The model under review builds one solid part; all positions refer to its coordinate system, in mm. Face numbers are marked on the shaded views. A direction names the side the tool comes from. Round coordinates to 2 decimals unless told otherwise and drop trailing zeros. Write each loop counter-clockwise with the first axis right and the second up, starting at its lowest first coordinate (ties: lowest second). Pieces come first, ordered by that corner, then holes. Notation, with made-up numbers: (-11, -29) - (-6, -29) arc R22 cw to (-6, 3) - close; hole circle Ø11 at (25, 5). An arc over 180 degrees is marked (long way). Use one line per item in the form item = value.
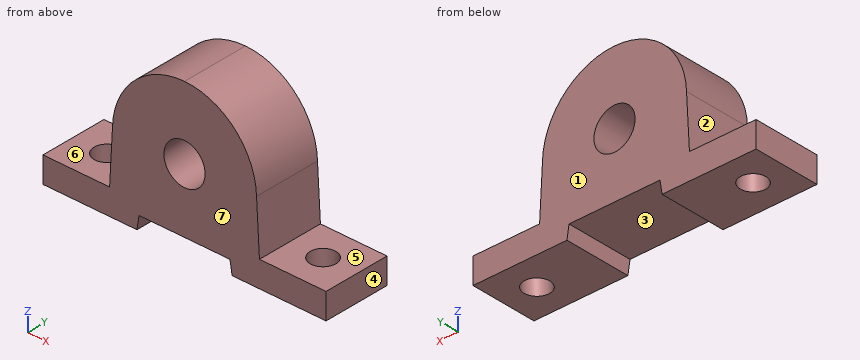
from build123d import *

# Parameters (mm, degrees)
PAD309_DEPTH      = 6.5
PAD309_DEPTH_BACK = 6.5
SKETCH722_R       = 2.5
POCKET253_DEPTH   = 100


with BuildPart() as part:
    # Sketch721 → Pad309 (new body, two sides)
    with BuildSketch(Plane.XZ) as pad309_sk:
        with BuildLine():
            ThreePointArc((13.993934, 15.412077), (9.752716, 25.04413), (0, 29))
            Line((0, 29), (0, 19))
            ThreePointArc((0, 11), (4, 15), (0, 19))
            Line((0, 11), (0, 2.582699))
            Line((8.836548, 2.582699), (0, 2.582699))
            Line((9.246055, 0), (8.836548, 2.582699))
            Line((27.5, 0), (9.246055, 0))
            Line((27.5, 5), (27.5, 0))
            Line((14.559493, 5), (27.5, 5))
            Line((13.993934, 15.412077), (14.559493, 5))
        make_face()
    pad309 = extrude(amount=PAD309_DEPTH) + extrude(pad309_sk.sketch, amount=-PAD309_DEPTH_BACK)

    # Mirrored001: Pad309 across Sketch721 V_Axis
    add(pad309.mirror(Plane(origin=(0, 0, 0), x_dir=(0, -1, 0), z_dir=(1, 0, 0))))

    # Sketch722 (on Face4 of Mirrored001) → Pocket253 (cut)
    with BuildSketch(Plane(origin=(0, 0, 5), x_dir=(-1, 0, 0), z_dir=(0, 0, 1))):
        with Locations((21, 0)):
            Circle(SKETCH722_R)
        with Locations((-21, 0)):
            Circle(SKETCH722_R)
    extrude(amount=-POCKET253_DEPTH, mode=Mode.SUBTRACT)


solid = part.part
(1) Add section C-C on z = 14.25. Write out the cut boundary in (x, y).
Geometry results:
outline = (-14.06, -6.5) - (-3.93, -6.5) - (-3.93, 6.5) - (-14.06, 6.5) - close; (3.93, -6.5) - (14.06, -6.5) - (14.06, 6.5) - (3.93, 6.5) - close
(2) The part is to be moulded in two halves that separate along X. For the marked faces 1, 2, 3 and 4, say which applies: +X half, -X half, draft (parallel to the pull), parting line (faces both ways), or undercut.
Geometry results:
face_1 = draft
face_2 = -X half
face_3 = undercut
face_4 = +X half
(3) Insertion check: P1, Ø2, axis at x = -7, y = 0, coming from the -Z side; P2, Ø4, axis at x = -18.5, y = 3, coming from the +Z side; P3, Ø1, axis at x = -3, y = -3.5, coming from the +Z side (3 decimals); P4, Ø3, axis at x = -21, y = 0, coming from the -Z side. Each pin has a flat end and moves straight along its axis. Give the tip position at first contact, or say it passes through.
Geometry results:
P1 = 2.58
P2 = 5
P3 = 28.775
P4 = through
(4) Add section B-B on x = -21. Write out the cut boundary in (y, z).
Geometry results:
outline = (-6.5, 0) - (-2.5, 0) - (-2.5, 5) - (-6.5, 5) - close; (2.5, 0) - (6.5, 0) - (6.5, 5) - (2.5, 5) - close
(5) To check wall thickness, follow L1, parallel to X at y = 0, z = 3.45; L2, parallel to Y at x = -21, z = 2.5; L3, parallel to X at y = 0, z = 1.9. State the ranges of each line that lie inside material, in increasing order.
Geometry results:
L1 = -27.5 to -23.5, -18.5 to 18.5, 23.5 to 27.5
L2 = -6.5 to -2.5, 2.5 to 6.5
L3 = -27.5 to -23.5, -18.5 to -8.94, 8.94 to 18.5, 23.5 to 27.5
(6) Add section D-D on y = 4. Write out the cut boundary in (x, z).
Geometry results:
outline = (-27.5, 0) - (-9.25, 0) - (-8.84, 2.58) - (8.84, 2.58) - (9.25, 0) - (27.5, 0) - (27.5, 5) - (14.56, 5) - (13.99, 15.41) arc R14 ccw to (0, 29) arc R14 ccw to (-13.99, 15.41) - (-14.56, 5) - (-27.5, 5) - close; hole circle Ø8 at (0, 15)
(7) Machinability: for the marked faces 5, 6 and 7, which of the approach directions +Z, -Z, +X, -X, +Y, -Y give a long, thin tool a straight path to every point of the face, cutting with its end or side? Answer none if there is none.
Geometry results:
face_5 = +Z, +X, +Y, -Y
face_6 = +Z, -X, +Y, -Y
face_7 = +Z, -Z, +X, -X, -Y
(8) Add section A-A on y = 0. Write out the cut boundary in (x, z), then the cut area to 3 significant figures.
Geometry results:
outline = (-27.5, 0) - (-23.5, 0) - (-23.5, 5) - (-27.5, 5) - close; (-18.5, 0) - (-9.25, 0) - (-8.84, 2.58) - (8.84, 2.58) - (9.25, 0) - (18.5, 0) - (18.5, 5) - (14.56, 5) - (13.99, 15.41) arc R14 ccw to (0, 29) arc R14 ccw to (-13.99, 15.41) - (-14.56, 5) - (-18.5, 5) - close; (23.5, 0) - (27.5, 0) - (27.5, 5) - (23.5, 5) - close; hole circle Ø8 at (0, 15)
area = 722 mm2
